from build123d import *

# Parameters (mm, degrees)
CROQUIS1_W              = 200
CROQUIS1_H              = 235
SALIENTE_EXTRUIR1_DEPTH = 235
CROQUIS2_W              = 49
CROQUIS2_H              = 49
SALIENTE_EXTRUIR2_DEPTH = 49


with BuildPart() as part:
    # Croquis1 → Saliente-Extruir1 (new body)
    with BuildSketch(Plane.XY):
        Rectangle(CROQUIS1_W, CROQUIS1_H)
    extrude(amount=SALIENTE_EXTRUIR1_DEPTH)

    # Croquis2 → Saliente-Extruir2 (add)
    with BuildSketch(Plane(origin=(100, 0, 0), x_dir=(0, 0, -1), z_dir=(1, 0, 0))):
        with Locations((-117.5, 0)):
            Rectangle(CROQUIS2_W, CROQUIS2_H)
    extrude(amount=SALIENTE_EXTRUIR2_DEPTH)


solid = part.part
Can you work these out from the model? Positions are in its coordinate system, mm. A direction names the side the tool comes from. Give positions to 0.01 mm unless a question says otherwise; leave off trailing zeros. Write each loop counter-clockwise with the first axis right and the second up, starting at its lowest first coordinate (ties: lowest second). Pieces come first, ordered by that corner, then holes. Notation, with made-up numbers: (75, 80.5) -> (132, 80.5) arc R13 cw to (132, 91.5) -> close; hole circle Ø2 at (62, 7). An arc over 180 degrees is marked (long way). Answer as a JSON object with one key per item and string values. Group by question number.
Item 1: Suppose I cut it at A-A (z = 99). Please give me the cut outline in (x, y), plus the area to 3 significant figures.
Item 2: Please list where this line runs through material, in increasing order: line 1 (X direction, y = -93.5, z = 220.5). Write a range as [from, to].
Item 3: Suppose I cut it at C-C (y = 38.5). Please give me the cut outline in (x, z), plus the area to 3 significant figures.
Item 4: Suppose I cut it at B-B (y = 3). Please give me the cut outline in (x, z), plus the area to 3 significant figures.
Item 5: For faces 1 (the face through (124, 0, 93)), 2 (the face through (-100, -2, 116)), 3 (the face through (124, 0, 142)), 4 (the face through (124, -24.5, 118)), 5 (the face through (124, 24.5, 118)), which set-ups out of +Z, -Z, +X, -X, +Y, -Y let a thin tool reach every point of the face, with its end or its side?
Item 6: I'm going to push flat-ended pins straight in: P1, Ø1.5, axis at y = 53.5, z = 58, coming from the +X side; P2, Ø14.5, axis at x = 125.5, z = 127.5, coming from the +Y side; P3, Ø14.5, axis at x = 114.5, z = 115, coming from the -Y side. Where does each tip first touch, or does it pass through?
Item 7: Suppose I cut it at D-D (z = 213). Please give me the cut outline in (x, y).
Findings:
{
 "1": {"outline": "(-100, -117.5) -> (100, -117.5) -> (100, -24.5) -> (149, -24.5) -> (149, 24.5) -> (100, 24.5) -> (100, 117.5) -> (-100, 117.5) -> close", "area": "49,400 mm²"},
 "2": {"line 1": "x = [-100, 100]"},
 "3": {"outline": "(-100, 0) -> (100, 0) -> (100, 235) -> (-100, 235) -> close", "area": "47,000 mm²"},
 "4": {"outline": "(-100, 0) -> (100, 0) -> (100, 93) -> (149, 93) -> (149, 142) -> (100, 142) -> (100, 235) -> (-100, 235) -> close", "area": "49,400 mm²"},
 "5": {"face 1": "-Z, +X, +Y, -Y", "face 2": "+Z, -Z, -X, +Y, -Y", "face 3": "+Z, +X, +Y, -Y", "face 4": "+Z, -Z, +X, -Y", "face 5": "+Z, -Z, +X, +Y"},
 "6": {"P1": "stops at x = 100", "P2": "stops at y = 24.5", "P3": "stops at y = -24.5"},
 "7": {"outline": "(-100, -117.5) -> (100, -117.5) -> (100, 117.5) -> (-100, 117.5) -> close"}
}
